The listing builds one solid part. Answer for the finished solid, in the listing's coordinates (mm). Give positions to 0.01 mm unless a question says otherwise; leave off trailing zeros. Write each loop counter-clockwise with the first axis right and the second up, starting at its lowest first coordinate (ties: lowest second). Pieces come first, ordered by that corner, then holes. Notation, with made-up numbers: (-14.75, 6) - (23.25, 6) arc R26 ccw to (23.25, 39) - close; hole circle Ø10 at (31, 6). An arc over 180 degrees is marked (long way). One line per question, with ' | ' between items. Start each with the question number.
1. Given P1, Ø6, axis at y = 52, z = 0.5, coming from the -X side; P2, Ø1, axis at x = -15.5, y = 58.5, coming from the +Z side, each flat-ended and moving along its own axis, determine where each tip first touches the part or whether it passes through.
2. A cutting plane is placed at B-B (z = -5.5). Determine the outline of the cut face in (x, y).
3. A cutting plane is placed at A-A (z = 0.25). Determine the outline of the cut face in (x, y), then the cut area to 3 significant figures.
4. Find the intervals of material crossed by L1, parallel to Y at x = -15.5, z = 3.75; L2, parallel to Y at x = -15.5, z = -2; L3, parallel to Y at x = -15.9, z = 3.25, in increasing order. Write a range as from..to.
```python
from build123d import *

# Parameters (mm, degrees)
SKETCH1_R                = 1
BOSS_EXTRUDE1_DEPTH      = 59.28
CUT_EXTRUDE1_DEPTH       = 59.28
SKETCH3_R                = 1
BOSS_EXTRUDE2_DEPTH      = 5
BOSS_EXTRUDE2_DEPTH_BACK = 3
BOSS_EXTRUDE3_START      = -2.5
SKETCH4_R                = 1
BOSS_EXTRUDE3_DEPTH      = 5
CUT_EXTRUDE2_DEPTH       = 15
SKETCH6_R                = 1
BOSS_EXTRUDE4_DEPTH      = 13


with BuildPart() as part:
    # Sketch1 → Boss-Extrude1 (new body)
    with BuildSketch(Plane(origin=(0, 0, 0), x_dir=(1, 0, 0), z_dir=(0, 1, 0))):
        with Locations((-15.419703787, 2.701939454)):
            Circle(SKETCH1_R)
    extrude(amount=BOSS_EXTRUDE1_DEPTH)

    # Sketch2 → Cut-Extrude1 (cut)
    with BuildSketch(Plane.XY):
        with BuildLine():
            Line((-16.419703787, 59.28), (-16.419703787, 58.28))
            ThreePointArc((-16.419703787, 58.28), (-16.126810568, 58.987106781), (-15.419703787, 59.28))
            Line((-15.419703787, 59.28), (-16.419703787, 59.28))
        make_face()
        with BuildLine():
            ThreePointArc((-15.419703787, 59.28), (-14.712597006, 58.987106781), (-14.419703787, 58.28))
            Line((-14.419703787, 58.28), (-14.419703787, 59.28))
            Line((-14.419703787, 59.28), (-15.419703787, 59.28))
        make_face()
    extrude(amount=-CUT_EXTRUDE1_DEPTH, mode=Mode.SUBTRACT)

    # Sketch3 → Boss-Extrude2 (add, two sides)
    with BuildSketch(Plane.XY) as boss_extrude2_sk:
        with Locations((-15.419703787, 58.28)):
            Circle(SKETCH3_R)
    extrude(amount=BOSS_EXTRUDE2_DEPTH)
    extrude(boss_extrude2_sk.sketch, amount=-BOSS_EXTRUDE2_DEPTH_BACK)

    # Sketch4 → Boss-Extrude3 (add)
    with BuildSketch(Plane.XY.offset(BOSS_EXTRUDE3_START)):
        with Locations((-15.419703787, 1)):
            Circle(SKETCH4_R)
    extrude(amount=-BOSS_EXTRUDE3_DEPTH)

    # Sketch5 → Cut-Extrude2 (cut)
    with BuildSketch(Plane(origin=(0, 0, -7.5), x_dir=(-1, 0, 0), z_dir=(0, 0, -1))):
        with BuildLine():
            ThreePointArc((15.419703787, 0), (14.712597006, 0.292893219), (14.419703787, 1))
            Line((14.419703787, 1), (14.419703787, 0))
            Line((14.419703787, 0), (15.419703787, 0))
        make_face()
        with BuildLine():
            Line((16.419703787, 0), (16.419703787, 1))
            ThreePointArc((16.419703787, 1), (16.126810568, 0.292893219), (15.419703787, 0))
            Line((15.419703787, 0), (16.419703787, 0))
        make_face()
    extrude(amount=-CUT_EXTRUDE2_DEPTH, mode=Mode.SUBTRACT)

    # Sketch6 → Boss-Extrude4 (add)
    with BuildSketch(Plane(origin=(0, 0, -7.5), x_dir=(-1, 0, 0), z_dir=(0, 0, -1))):
        with Locations((15.419703787, 1)):
            Circle(SKETCH6_R)
    extrude(amount=-BOSS_EXTRUDE4_DEPTH)


solid = part.part
```
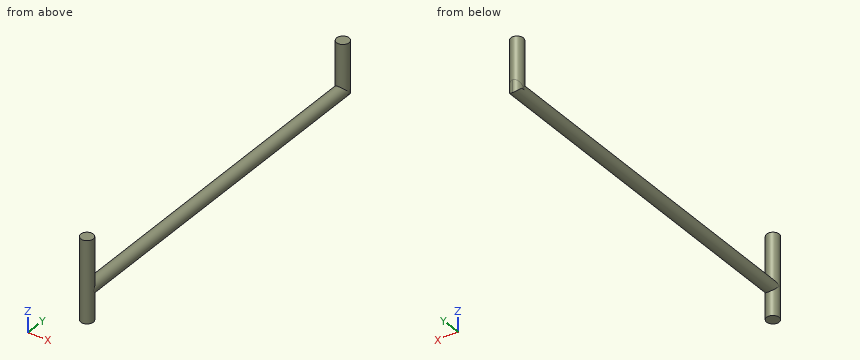
Determined:
1) P1: x = -16.4 | P2: z = 5
2) outline: circle Ø2 at (-15.42, 1)
3) outline: circle Ø2 at (-15.42, 1); circle Ø2 at (-15.42, 58.28) | area: 6.28 mm2
4) L1: 0..2, 57.28..59.28 | L2: 0..59.28 | L3: 0.12..1.88, 57.4..59.16
